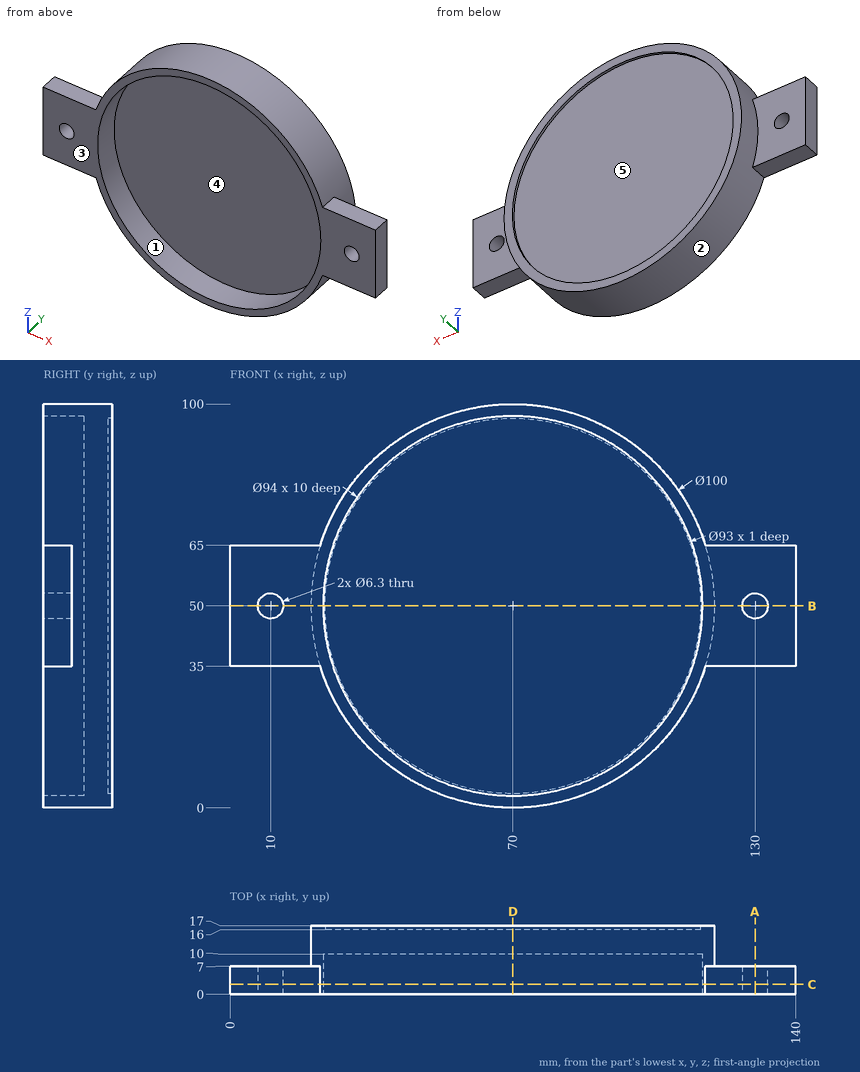
Source: three-view drawing plus pictorial views. Frame: mm from the lowest corner of the part. A direction names the side the tool comes from. Coordinates: 2 decimals unless noted, no trailing zeros. Loops run counter-clockwise (first coordinate to the right, second up) from the corner with the lowest first, then second, coordinate; pieces in that order, holes last. Notation, with made-up numbers: M 20.5,39 L 65.5,39 A15 cw 65.5,57 Z; hole C 82.5,83 d7. An arc over 180 degrees is marked long. Use CSV: the item, a comma, the result in double quotes.
(1) Cut plane C-C on y = 2.5. Return loops of the section in (x, z).
Answers follow:
outline,"M 0,35 L 22.3,35 A50 ccw 117.7,35 L 140,35 L 140,65 L 117.7,65 A50 ccw 22.3,65 L 0,65 Z; hole C 10,50 d6.3; hole C 70,50 d94; hole C 130,50 d6.3"
(2) Reachability of the marked faces 4 and 5 from +Z, -Z, +X, -X, +Y, -Y: full face, straight path, thin tool, end or side. Return the list, or none.
Answers follow:
face 4,"-Y"
face 5,"+Y"
(3) Contact query for flat-ended pins moving along their axis: pin 1 (5 mm diameter, centred on x = 130, z = 50, fed in from +Y); pin 2 (10 mm diameter, centred on y = 8.5, z = 83.5, fed in from +X); pin 3 (18 mm diameter, centred on x = 134, z = 49.5, fed in from +Y); pin 4 (6 mm diameter, centred on x = 102, y = 8, fed in from -Z). Output: stop coordinate, or through.
Answers follow:
pin 1,"through"
pin 2,"x = 111.08"
pin 3,"y = 7"
pin 4,"z = 9.27"
(4) Cut plane B-B on z = 50. Return loops of the section in (x, y).
Answers follow:
outline,"M 0,0 L 6.85,0 L 6.85,7 L 0,7 Z; M 13.15,0 L 23,0 L 23,10 L 117,10 L 117,0 L 126.85,0 L 126.85,7 L 120,7 L 120,17 L 116.5,17 L 116.5,16 L 23.5,16 L 23.5,17 L 20,17 L 20,7 L 13.15,7 Z; M 133.15,0 L 140,0 L 140,7 L 133.15,7 Z"
(5) Line query: line 1 (Z direction, x = 70, y = 3); line 2 (Z direction, x = 70, y = 16.6); line 3 (Y direction, x = 103, z = 22.5). Output: solid intervals per line, ascending. Write a range as [from, to].
Answers follow:
line 1,"[0, 3], [97, 100]"
line 2,"[0, 3.5], [96.5, 100]"
line 3,"[10, 16]"
(6) Cut plane D-D on x = 70. Return loops of the section in (y, z), and give its area (3 significant figures).
Answers follow:
outline,"M 0,0 L 17,0 L 17,3.5 L 16,3.5 L 16,96.5 L 17,96.5 L 17,100 L 0,100 L 0,97 L 10,97 L 10,3 L 0,3 Z"
area,"667 mm²"
(7) Cut plane A-A on x = 130. Return loops of the section in (y, z).
Answers follow:
outline,"M 0,35 L 7,35 L 7,46.85 L 0,46.85 Z; M 0,53.15 L 7,53.15 L 7,65 L 0,65 Z"
(8) Draft query along X for the marked faces 1, 2 and 3. Return one class per face: pulls with the +X half, pulls with the -X half, needs draft (parallel to the pull), parting line crosses it, or undercut.
Answers follow:
face 1,"undercut"
face 2,"parting line crosses it"
face 3,"needs draft"
